For this review, use the dimensioned drawing (mm, ordinates from the lowest corner) and the shaded views. A direction names the side the tool comes from. Round coordinates to 2 decimals unless told otherwise and drop trailing zeros. Loops run counter-clockwise (first coordinate to the right, second up) from the corner with the lowest first, then second, coordinate; pieces in that order, holes last. Notation, with made-up numbers: M 36,-23.5 L 54,-23.5 A17 cw 54,-0.5 Z; hole C 42.25,59 d9. An arc over 180 degrees is marked long. One line per item, written item: value. Start each with the question number.
Item 1: We need section B-B (y = 3.25). Write out the cut boundary in (x, z).
Item 2: For line 1 along Z through (x, y) = (3.75, 1.75); line 2 along Y through (x, z) = (1, 36) (1 decimal); line 3 along X through (y, z) = (5.75, 59), list the stretches that pass through material, from the lowest coordinate up.
Item 3: We need section A-A (x = 7.25). Write out the cut boundary in (y, z) (1 decimal), then the cut area to 3 significant figures.
Item 4: We need section D-D (x = 1.25). Write out the cut boundary in (y, z).
Item 5: For the marked faces 1, 2 and 3, list the 3-axis set-ups (+Z, -Z, +X, -X, +Y, -Y) from which the entire face can be reached by the end or side of a thin tool; tool diameter is ignored.
Item 6: Clearance check with flat-ended pins moving along their axes: pin 1 (1 mm diameter, centred on y = 11, z = 63, fed in from -X) (1 decimal); pin 2 (1.5 mm diameter, centred on y = 13.5, z = 13, fed in from +X); pin 3 (1.5 mm diameter, centred on x = 3, z = 25.5, fed in from +Y). State where each tip first meets the part, or that it passes through.
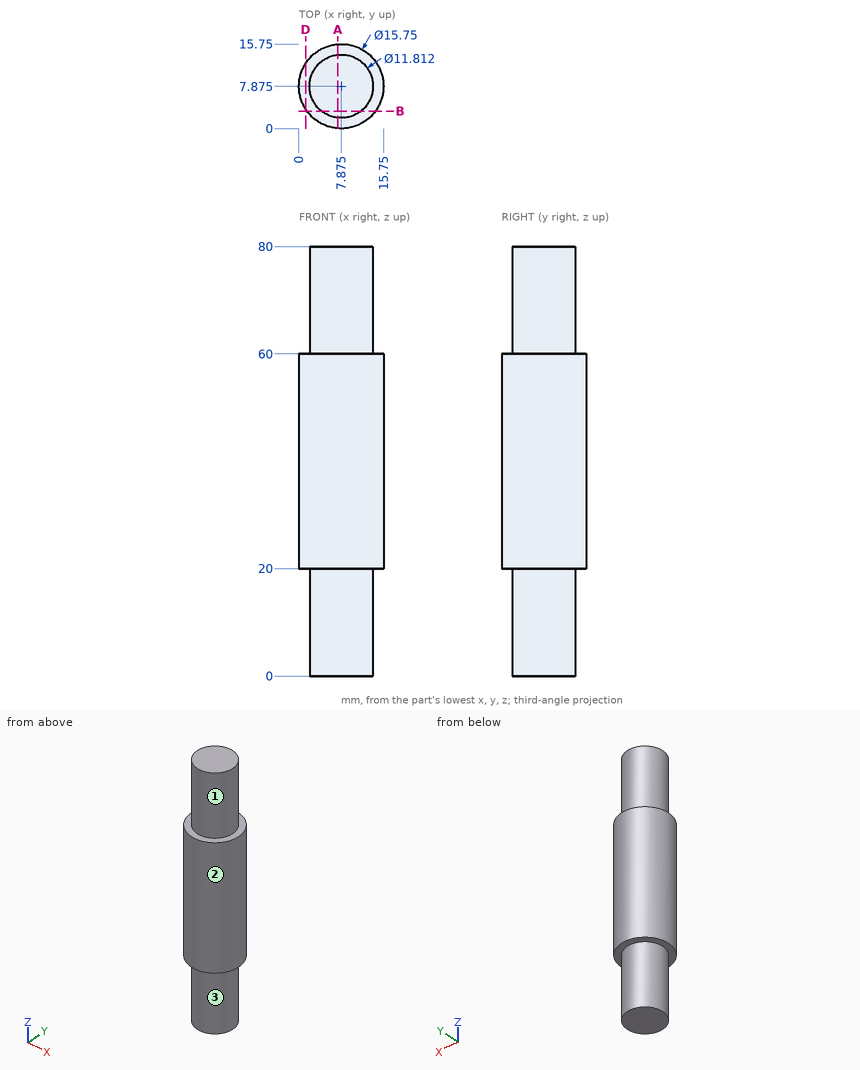
A:
1. outline: M 1.5,20 L 4.2,20 L 4.2,0 L 11.55,0 L 11.55,20 L 14.25,20 L 14.25,60 L 11.55,60 L 11.55,80 L 4.2,80 L 4.2,60 L 1.5,60 Z
2. line 1: 20 to 60
2. line 2: 4 to 11.7
2. line 3: 0.29 to 15.46
3. outline: M 0,20 L 2,20 L 2,0 L 13.7,0 L 13.7,20 L 15.7,20 L 15.7,60 L 13.7,60 L 13.7,80 L 2,80 L 2,60 L 0,60 Z
3. area: 1,100 mm2
4. outline: M 3.62,20 L 12.13,20 L 12.13,60 L 3.62,60 Z
5. face 1: +Z
5. face 2: +Z, -Z
5. face 3: -Z
6. pin 1: x = 2.6
6. pin 2: x = 11.21
6. pin 3: y = 14.58
